```python
from build123d import *

# Parameters (mm, degrees)
SKETCH032_W     = 40
SKETCH032_H     = 40
SKETCH032_R     = 2
PAD018_DEPTH    = 2
SKETCH033_W     = 32
SKETCH033_H     = 32
SKETCH033_R     = 2
PAD019_DEPTH    = 10
SKETCH034_R     = 2
POCKET013_DEPTH = 8
SKETCH035_R     = 2
POCKET014_DEPTH = 8
SKETCH039_R     = 2
POCKET015_DEPTH = 8


with BuildPart() as part:
    # Sketch032 → Pad018 (new body)
    with BuildSketch(Plane.XZ):
        with Locations((0, 20)):
            Rectangle(SKETCH032_W, SKETCH032_H)
        with Locations((-12.5, 7.5)):
            Circle(SKETCH032_R, mode=Mode.SUBTRACT)
        with Locations((-12.5, 32.5)):
            Circle(SKETCH032_R, mode=Mode.SUBTRACT)
        with Locations((12.5, 32.5)):
            Circle(SKETCH032_R, mode=Mode.SUBTRACT)
        with Locations((12.5, 7.5)):
            Circle(SKETCH032_R, mode=Mode.SUBTRACT)
    extrude(amount=-PAD018_DEPTH)

    # Sketch033 (on Face9 of Pad018) → Pad019 (join)
    with BuildSketch(Plane.XZ):
        with Locations((0, 20)):
            Rectangle(SKETCH033_W, SKETCH033_H)
        with Locations((-12.5, 32.5)):
            Circle(SKETCH033_R, mode=Mode.SUBTRACT)
        with Locations((12.5, 32.5)):
            Circle(SKETCH033_R, mode=Mode.SUBTRACT)
        with Locations((-12.5, 7.5)):
            Circle(SKETCH033_R, mode=Mode.SUBTRACT)
        with Locations((12.5, 7.5)):
            Circle(SKETCH033_R, mode=Mode.SUBTRACT)
    extrude(amount=PAD019_DEPTH)

    # Sketch034 (on Face10 of Pad019) → Pocket013 (cut)
    with BuildSketch(Plane(origin=(-16, 0, 0), x_dir=(0, 0, -1), z_dir=(-1, 0, 0))):
        with Locations((-28, 5)):
            Circle(SKETCH034_R)
        with Locations((-12, 5)):
            Circle(SKETCH034_R)
    extrude(amount=-POCKET013_DEPTH, mode=Mode.SUBTRACT)

    # Sketch035 (on Face7 of Pocket013) → Pocket014 (cut)
    with BuildSketch(Plane(origin=(0, 0, 36), x_dir=(-1, 0, 0), z_dir=(0, 0, 1))):
        with Locations((-8, 5)):
            Circle(SKETCH035_R)
        with Locations((8, 5)):
            Circle(SKETCH035_R)
    extrude(amount=-POCKET014_DEPTH, mode=Mode.SUBTRACT)

    # Sketch039 (on Face8 of Pocket014) → Pocket015 (cut)
    with BuildSketch(Plane(origin=(16, 0, 0), x_dir=(0, 0, 1), z_dir=(1, 0, 0))):
        with Locations((12, 5)):
            Circle(SKETCH039_R)
        with Locations((28, 5)):
            Circle(SKETCH039_R)
    extrude(amount=-POCKET015_DEPTH, mode=Mode.SUBTRACT)


solid = part.part
```
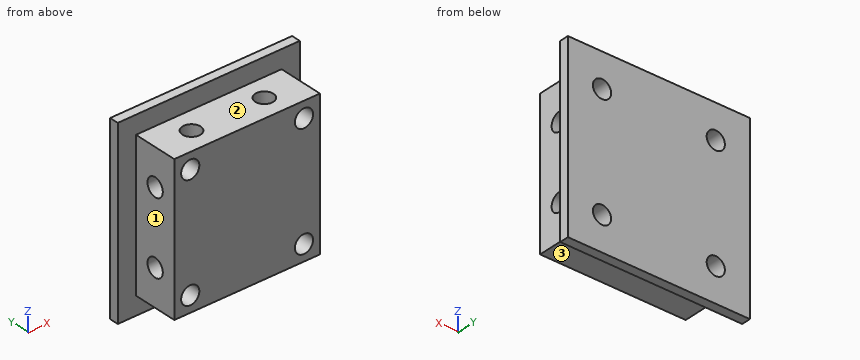
Input: part model. Units: mm. Frame: model coordinates. Face numbers are marked on the shaded views. A direction names the side the tool comes from. Coordinates: 2 decimals unless noted, no trailing zeros. Loops run counter-clockwise (first coordinate to the right, second up) from the corner with the lowest first, then second, coordinate; pieces in that order, holes last.
Q1. Section D-D, the plane z = 12. Return the cut outline in (x, y).
Results are:
outline: (-20, 0) - (-16, 0) - (-16, -3) - (-8, -3) - (-8, -7) - (-16, -7) - (-16, -10) - (16, -10) - (16, -7) - (8, -7) - (8, -3) - (16, -3) - (16, 0) - (20, 0) - (20, 2) - (-20, 2) - close
Q2. Set-up query: the marked faces 1, 2 and 3. Return all of +Z, -Z, +X, -X, +Y, -Y with unobstructed straight access to the full face (end or side cutting, diameter ignored); none if empty.
Results are:
face 1: +Z, -Z, -X, -Y
face 2: +Z, +X, -X, -Y
face 3: -Z, +X, -X, -Y
Q3. Section A-A, the plane y = -5. Give the number of separate pieces and of enclosed holes in the cut face, and give its area (3 significant figures).
Results are:
separate pieces: 3
enclosed holes: 4
area: 790 mm2
Q4. Section B-B, the plane x = 12.5. Return the cut outline in (y, z).
Results are:
outline: (-10, 4) - (0, 4) - (0, 0) - (2, 0) - (2, 5.5) - (-10, 5.5) - close; (-10, 9.5) - (2, 9.5) - (2, 30.5) - (-10, 30.5) - close; (-10, 34.5) - (2, 34.5) - (2, 40) - (0, 40) - (0, 36) - (-10, 36) - close; hole circle Ø4 at (-5, 12); hole circle Ø4 at (-5, 28)
Q5. Section C-C, the plane z = 32.5. Return the cut outline in (x, y), and give its area (3 significant figures).
Results are:
outline: (-20, 0) - (-16, 0) - (-16, -10) - (-14.5, -10) - (-14.5, 2) - (-20, 2) - close; (-10.5, -10) - (10.5, -10) - (10.5, 2) - (-10.5, 2) - close; (14.5, -10) - (16, -10) - (16, 0) - (20, 0) - (20, 2) - (14.5, 2) - close; hole circle Ø4 at (-8, -5); hole circle Ø4 at (8, -5)
area: 279 mm2
Q6. Line query: line 1 along Z through (x, y) = (14.75, -5); line 2 along X through (y, z) = (-5.25, 32); line 3 along X through (y, z) = (-5, 32.75). Output: solid intervals per line, ascending.
Results are:
line 1: z = 4 to 10, 14 to 26, 30 to 36
line 2: x = -16 to -14.44, -10.56 to -9.98, -6.02 to 6.02, 9.98 to 10.56, 14.44 to 16
line 3: x = -16 to -14.48, -10.52 to -10, -6 to 6, 10 to 10.52, 14.48 to 16
Q7. Contact query for flat-ended pins moving along their axis: pin 1 (2.5 mm diameter, centred on x = 12.5, z = 7.5, fed in from +Y); pin 2 (5 mm diameter, centred on x = 4.5, y = -4.5, fed in from +Z); pin 3 (1.5 mm diameter, centred on x = -8, y = -4, fed in from -Z); pin 4 (1 mm diameter, centred on y = -5, z = 27, fed in from +X). Output: stop coordinate, or through.
Results are:
pin 1: passes through
pin 2: stops at z = 36
pin 3: stops at z = 4
pin 4: stops at x = 8
